Input: part model. Units: mm. Frame: model coordinates. A direction names the side the tool comes from. Round coordinates to 2 decimals unless told otherwise and drop trailing zeros. Loops run counter-clockwise (first coordinate to the right, second up) from the corner with the lowest first, then second, coordinate; pieces in that order, holes last. Notation, with made-up numbers: (59.5, 33.5) -> (79.5, 33.5) arc R21 cw to (79.5, 51.5) -> close; hole circle Ø5 at (-28.75, 6). An arc over 180 degrees is marked (long way). Answer in a Markdown table with one row per item. Add a question column.
Q1. Section B-B, the plane x = -17. Output: boundary loops of the cut face in (y, z).
Q2. Section D-D, the plane z = -1.5. Give the number of separate pieces and of enclosed holes in the cut face, and give its area (3 significant figures).
Q3. Section C-C, the plane y = 30. Output: boundary loops of the cut face in (x, z), and give its area (3 significant figures).
Q4. Ray query, L1, parallel to X at y = 11.5, z = -8; L2, parallel to Y at x = -13.5, z = -4.5; L3, parallel to Y at x = 39, z = -6. Return the intervals inside material, ascending. Write a range as from..to.
Q5. Reachability of faces 4 (the face through (-34.83, -30.16, -7.5)), 5 (the face through (-1, 19, -10)), 6 (the face through (20, 0, -5)) from +Z, -Z, +X, -X, +Y, -Y: full face, straight path, thin tool, end or side. Return the list, or none.
Q6. Section A-A, the plane y = -0.5. Output: boundary loops of the cut face in (x, z), and give its area (3 significant figures).
Q7. Mould query, pull axis X, two halves, no side actions, for faces 1 (the face through (1, 40.5, -5)), 2 (the face through (50, -1, -5)), 3 (the face through (-20, 0, -5)). Classes: pulls with the +X half, pulls with the -X half, needs draft (parallel to the pull), parting line crosses it, or undercut.
```python
from build123d import *

# Parameters (mm, degrees)
F0_W     = 100
F0_H     = 60
F0_W_2   = 40
F0_H_2   = 30
F1_DEPTH = 10
F2_DEPTH = 10.001


with BuildPart() as f1:
    # F0 (on Top) → F1 (new body)
    with BuildSketch(Plane.XY):
        Polygon((50, -35), (50, -30), (-50, -30), (-50, -35), (-47, -35), (-47, -37.5), (-23, -37.5), (-23, -35), (0, -35), (23, -35), (23, -37.5), (47, -37.5), (47, -35), align=None)
        Rectangle(F0_W, F0_H)
        Rectangle(F0_W_2, F0_H_2, mode=Mode.SUBTRACT)
        Polygon((50, 30), (50, 35), (47, 35), (47, 37.5), (23, 37.5), (23, 35), (0, 35), (-23, 35), (-23, 37.5), (-47, 37.5), (-47, 35), (-50, 35), (-50, 30), align=None)
        Polygon((50, -40.5), (50, -35), (47, -35), (47, -37.5), (23, -37.5), (23, -35), (0, -35), (-23, -35), (-23, -37.5), (-47, -37.5), (-47, -35), (-50, -35), (-50, -40.5), align=None)
        Polygon((50, 35), (50, 40.5), (-50, 40.5), (-50, 35), (-47, 35), (-47, 37.5), (-23, 37.5), (-23, 35), (0, 35), (23, 35), (23, 37.5), (47, 37.5), (47, 35), align=None)
        Rectangle(F0_W_2, F0_H_2)
    extrude(amount=-F1_DEPTH)

    # F0 (on Top) → F2 (cut, through all)
    with BuildSketch(Plane.XY):
        Rectangle(F0_W_2, F0_H_2)
    extrude(amount=-F2_DEPTH, mode=Mode.SUBTRACT)

    # F0 (on Top) → F3 (revolve, cut)
    with BuildSketch(Plane.XY):
        Polygon((50, 30), (50, 35), (47, 35), (47, 37.5), (23, 37.5), (23, 35), (0, 35), (-23, 35), (-23, 37.5), (-47, 37.5), (-47, 35), (-50, 35), (-50, 30), align=None)
    revolve(axis=Axis((0, 30, 0), (1, 0, 0)), mode=Mode.SUBTRACT)

    # F0 (on Top) → F4 (revolve, cut)
    with BuildSketch(Plane.XY):
        Polygon((50, -35), (50, -30), (-50, -30), (-50, -35), (-47, -35), (-47, -37.5), (-23, -37.5), (-23, -35), (0, -35), (23, -35), (23, -37.5), (47, -37.5), (47, -35), align=None)
    revolve(axis=Axis((0, -30, 0), (1, 0, 0)), mode=Mode.SUBTRACT)


solid = f1.part
```
Answer block:
| question | item | result |
|---|---|---|
| 1 | outline | (-40.5, -10) -> (-15, -10) -> (-15, 0) -> (-25, 0) arc R5 cw to (-35, 0) -> (-40.5, 0) -> close; (15, -10) -> (40.5, -10) -> (40.5, 0) -> (35, 0) arc R5 cw to (25, 0) -> (15, 0) -> close |
| 2 | separate pieces | 3 |
| 2 | enclosed holes | 1 |
| 2 | area | 4,500 mm^2 |
| 3 | outline | (-50, -10) -> (50, -10) -> (50, -5) -> (47, -5) -> (47, -7.5) -> (23, -7.5) -> (23, -5) -> (-23, -5) -> (-23, -7.5) -> (-47, -7.5) -> (-47, -5) -> (-50, -5) -> close |
| 3 | area | 380 mm^2 |
| 4 | L1 | -50..-20, 20..50 |
| 4 | L2 | -40.5..-32.18, -27.82..-15, 15..27.82, 32.18..40.5 |
| 4 | L3 | -40.5..-34.5, -25.5..25.5, 34.5..40.5 |
| 5 | face 4 | +Z |
| 5 | face 5 | -Z, +X, -X, +Y, -Y |
| 5 | face 6 | +Z, -Z |
| 6 | outline | (-50, -10) -> (-20, -10) -> (-20, 0) -> (-50, 0) -> close; (20, -10) -> (50, -10) -> (50, 0) -> (20, 0) -> close |
| 6 | area | 600 mm^2 |
| 7 | face 1 | needs draft |
| 7 | face 2 | pulls with the +X half |
| 7 | face 3 | undercut |
